Geometry check sheet. Reference: the model listing, model coordinates, mm. Face numbers are marked on the shaded views. A direction names the side the tool comes from. Round coordinates to 2 decimals unless told otherwise and drop trailing zeros. Order: outer loops, then holes, each group sorted by start corner. A loop starts at its lowest first (then second) coordinate and runs counter-clockwise, first axis right, second up.
```python
from build123d import *

# Parameters (mm, degrees)
F1_DEPTH  = 34.925
F2_R      = 2.6162
F3_DEPTH  = 74.931
F4_R      = 2.6162
F5_DEPTH  = 74.931
F6_R      = 3.175
F7_DEPTH  = 74.931
F8_R      = 6.35
F9_DEPTH  = 49.53
F11_DEPTH = 22.86
F13_DEPTH = 2.54


with BuildPart() as f1:
    # F0 (on Top) → F1 (new body)
    with BuildSketch(Plane.XY):
        with BuildLine():
            ThreePointArc((-1.5875, -44.2945614354), (-31.002155354, -31.6764059262), (-44.2501607794, -2.54))
            Line((-44.2501607794, -2.54), (-60.325, -2.54))
            Line((-60.325, -2.54), (-60.325, -69.1896))
            Line((-60.325, -69.1896), (-50.165, -77.47))
            Line((-50.165, -77.47), (-1.5875, -77.47))
            Line((-1.5875, -77.47), (-1.5875, -44.2945614354))
        make_face()
        Polygon((-1.5875, -40.513), (-1.5875, -44.2945614354), (-1.5875, -77.47), (1.5875, -77.47), (1.5875, -44.2945614354), (1.5875, -40.513), align=None)
        with BuildLine():
            Line((1.5875, -44.2945614354), (1.5875, -77.47))
            Line((1.5875, -77.47), (50.165, -77.47))
            Line((50.165, -77.47), (60.325, -69.1896))
            Line((60.325, -69.1896), (60.325, -2.54))
            Line((60.325, -2.54), (44.2501607794, -2.54))
            ThreePointArc((44.2501607794, -2.54), (31.002155354, -31.6764059262), (1.5875, -44.2945614354))
        make_face()
    extrude(amount=F1_DEPTH)

    # F2 (on face) → F3 (cut, through all)
    with BuildSketch(Plane(origin=(0, -2.54, 0), x_dir=(-1, 0, 0), z_dir=(0, 1, 0))):
        with Locations((-52.2875803897, 9.525)):
            Circle(F2_R)
    extrude(amount=-F3_DEPTH, mode=Mode.SUBTRACT)

    # F4 (on face) → F5 (cut, through all)
    with BuildSketch(Plane(origin=(0, -2.54, 0), x_dir=(-1, 0, 0), z_dir=(0, 1, 0))):
        with Locations((52.2875803897, 9.525)):
            Circle(F4_R)
    extrude(amount=-F5_DEPTH, mode=Mode.SUBTRACT)

    # F6 (on face) → F7 (cut, through all)
    with BuildSketch(Plane.XZ.offset(77.47)):
        with Locations((-47.625, 25.4)):
            Circle(F6_R)
        with Locations((47.625, 25.4)):
            Circle(F6_R)
        with Locations((0, 25.4)):
            Circle(F6_R)
    extrude(amount=-F7_DEPTH, mode=Mode.SUBTRACT)

    # F8 (on face) → F9 (cut)
    with BuildSketch(Plane(origin=(0, -2.54, 0), x_dir=(-1, 0, 0), z_dir=(0, 1, 0))):
        with Locations((-47.625, 25.4)):
            Circle(F8_R)
        with Locations((0, 25.4)):
            Circle(F8_R)
        with Locations((47.625, 25.4)):
            Circle(F8_R)
    extrude(amount=-F9_DEPTH, mode=Mode.SUBTRACT)

    # F10 (on face) → F11 (cut)
    with BuildSketch(Plane.XZ.offset(77.47)):
        Polygon((-49.3546410222, 4.445), (-46.4217016547, 9.525), (-49.3546410222, 14.605), (-55.2205197572, 14.605), (-58.1534591247, 9.525), (-55.2205197572, 4.445), align=None)
        Polygon((49.3546410222, 14.605), (46.4217016547, 9.525), (49.3546410222, 4.445), (55.2205197572, 4.445), (58.1534591247, 9.525), (55.2205197572, 14.605), align=None)
    extrude(amount=-F11_DEPTH, mode=Mode.SUBTRACT)

    # F12 (on face) → F13 (join)
    with BuildSketch(Plane.XY.offset(34.925)):
        Polygon((-1.5875, -41.783), (-1.5875, -44.323), (1.5875, -44.2945614354), (1.5875, -41.783), align=None)
    extrude(amount=-F13_DEPTH)


solid = f1.part
```
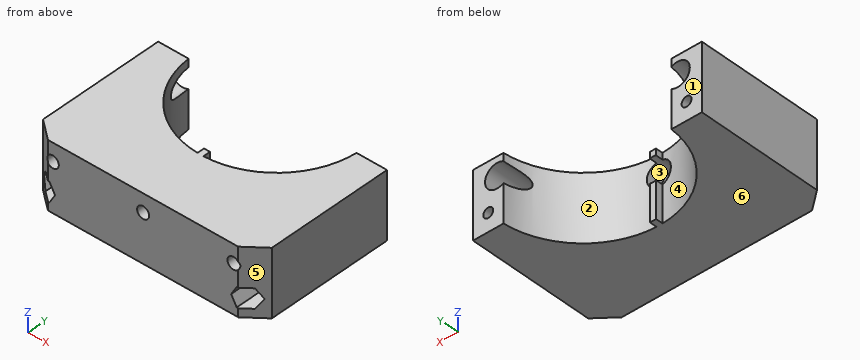
(1) Draft check along X on the marked faces 4, 5 and 6. Enter one of: released by +X, released by -X, zero draft, split by the parting line, or undercut.
Returned:
face 4: undercut
face 5: released by +X
face 6: zero draft
(2) Sectioned sample at D-D, the plane y = -27.5. Record the cut outline in (x, z) (3 decimals).
Returned:
outline: (-60.325, 0) - (-34.76, 0) - (-34.76, 34.925) - (-60.325, 34.925) - close; (34.76, 0) - (60.325, 0) - (60.325, 34.925) - (34.76, 34.925) - close; hole circle Ø5.232 at (-52.288, 9.525); hole circle Ø12.7 at (-47.625, 25.4); hole circle Ø12.7 at (47.625, 25.4); hole circle Ø5.232 at (52.288, 9.525)
(3) Sectioned sample at B-B, the plane y = -49. Record the cut outline in (x, z) (3 decimals), and give its area (3 significant figures).
Returned:
outline: (-60.325, 0) - (60.325, 0) - (60.325, 34.925) - (-60.325, 34.925) - close; hole circle Ø5.232 at (-52.288, 9.525); hole circle Ø12.7 at (-47.625, 25.4); hole circle Ø12.7 at (0, 25.4); hole circle Ø12.7 at (47.625, 25.4); hole circle Ø5.232 at (52.288, 9.525)
area: 3,790 mm2
(4) Sectioned sample at A-A, the plane x = 0. Record the cut outline in (y, z) (3 decimals), and give its area (3 significant figures).
Returned:
outline: (-77.47, 0) - (-40.513, 0) - (-40.513, 19.05) - (-52.07, 19.05) - (-52.07, 22.225) - (-77.47, 22.225) - close; (-77.47, 28.575) - (-52.07, 28.575) - (-52.07, 31.75) - (-40.513, 31.75) - (-40.513, 34.925) - (-77.47, 34.925) - close
area: 983 mm2
(5) Set-up check for the marked faces 1, 2 and 3: record each of +Z, -Z, +X, -X, +Y, -Y from which the full face is reachable in a straight line by a thin tool's end or side.
Returned:
face 1: +Z, -Z, +X, -X, +Y
face 2: +Z, -Z, +Y
face 3: +Y
(6) Material ranges on line 1 (X direction, y = -26.5, z = 25.4) (3 decimals); line 2 (Z direction, x = 47.5, y = -41) (3 decimals); line 3 (Z direction, x = -51.5, y = -28.5) (3 decimals), recorded low to high.
Returned:
line 1: x = -60.325 to -53.975, -41.275 to -35.529, 35.529 to 41.275, 53.975 to 60.325
line 2: z = 0 to 19.051, 31.749 to 34.925
line 3: z = 0 to 7.03, 12.02 to 20.369, 30.431 to 34.925
(7) Depth check by flat-ended pin: P1, Ø3.5, axis at x = -0.5, z = 33.5, coming from the +Y side; P2, Ø14, axis at x = 45, z = 22.5, coming from the +Y side; P3, Ø1, axis at x = -35, z = 15.5, coming from the +Y side; P4, Ø5, axis at x = -10, z = 29, coming from the +Y side. Enter the tip coordinate at first touch or a pass-through.
Returned:
P1: stops at y = -40.51
P2: stops at y = -2.54
P3: stops at y = -26.54
P4: stops at y = -42.52
(8) Sectioned sample at C-C, the plane z = 25.4. Record the cut outline in (x, y) (3 decimals).
Returned:
outline: (-60.325, -69.19) - (-50.8, -76.952) - (-50.8, -52.07) - (-53.975, -52.07) - (-53.975, -2.54) - (-60.325, -2.54) - close; (-44.45, -77.47) - (-3.175, -77.47) - (-3.175, -52.07) - (-6.35, -52.07) - (-6.35, -43.866) arc R44.323 cw to (-41.275, -16.152) - (-41.275, -52.07) - (-44.45, -52.07) - close; (3.175, -77.47) - (44.45, -77.47) - (44.45, -52.07) - (41.275, -52.07) - (41.275, -16.152) arc R44.323 cw to (6.35, -43.866) - (6.35, -52.07) - (3.175, -52.07) - close; (50.8, -76.952) - (60.325, -69.19) - (60.325, -2.54) - (53.975, -2.54) - (53.975, -52.07) - (50.8, -52.07) - close
